Design review of the part shown in the three views and the two pictorial views. Dimensions are in mm from the part's minimum x, y and z. A direction names the side the tool comes from. Coordinates: 2 decimals unless noted, no trailing zeros. Write each loop counter-clockwise with the first axis right and the second up, starting at its lowest first coordinate (ties: lowest second). Pieces come first, ordered by that corner, then holes.
Q1. For the marked faces 4 and 5, list the 3-axis set-ups (+Z, -Z, +X, -X, +Y, -Y) from which the entire face can be reached by the end or side of a thin tool; tool diameter is ignored.
Q2. The part is to be moulded in two halves that separate along Z. For the marked faces 1, 2 and 3, say which applies: released by +Z, released by -Z, zero draft, split by the parting line, or undercut.
Q3. Take a section at C-C, the plane x = 1.25. Write out the cut boundary in (y, z), plus the area to 4 significant figures.
Q4. For pin 1 Ø5 at (x, z) = (4.5, 19) entering from -Y; pin 2 Ø4 at (y, z) = (9.5, 27) entering from +X, all flat-tipped, find the tip position at first contact; note any pin that passes through.
Q5. Take a section at B-B, the plane y = 18.5. Write out the cut boundary in (x, z).
Q6. For L1, parallel to Z at x = 8.75, y = 38; L2, parallel to Y at x = 2.5, z = 2, list the stretches that pass through material, from the lowest coordinate up.
Q7. Take a section at A-A, the plane z = 27. Write out the cut boundary in (x, y).
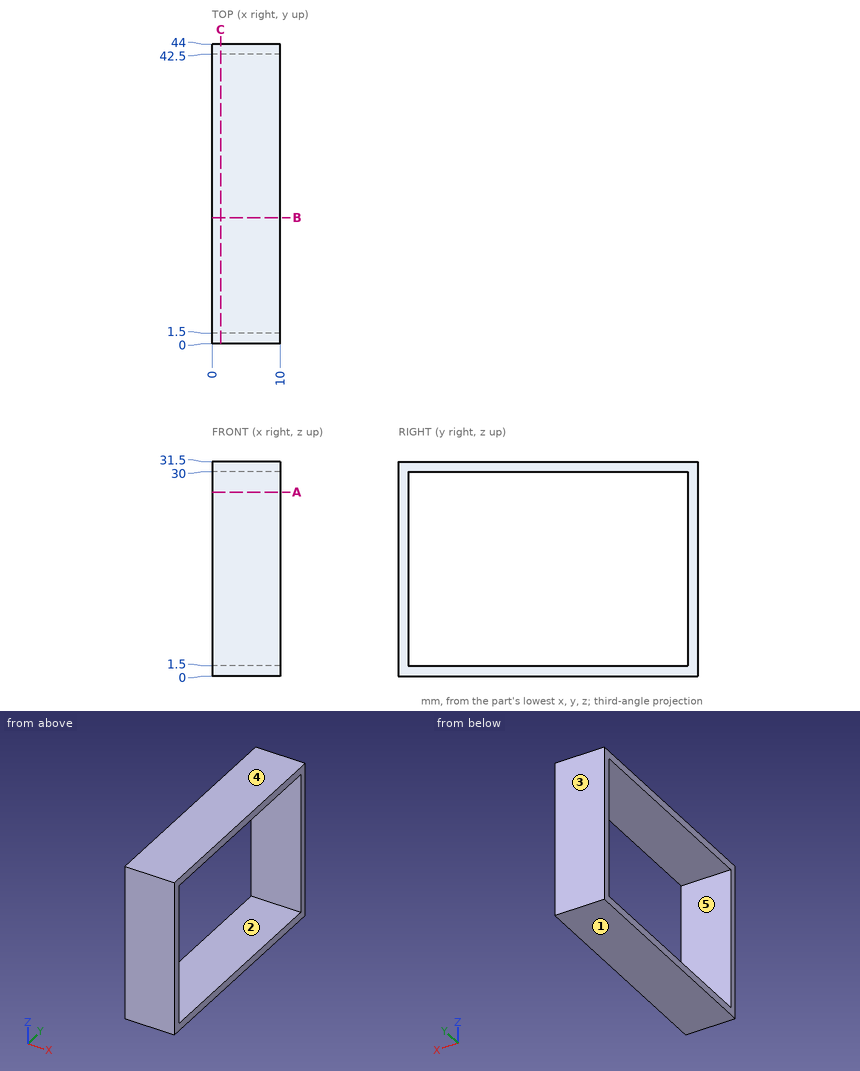
Responses:
1. face 4: +Z, +X, -X, +Y, -Y
1. face 5: +X, -X
2. face 1: released by -Z
2. face 2: undercut
2. face 3: zero draft
3. outline: (0, 0) - (44, 0) - (44, 31.5) - (0, 31.5) - close; hole (1.5, 1.5) - (42.5, 1.5) - (42.5, 30) - (1.5, 30) - close
3. area: 217.5 mm2
4. pin 1: stops at y = 0
4. pin 2: passes through
5. outline: (0, 0) - (10, 0) - (10, 1.5) - (0, 1.5) - close; (0, 30) - (10, 30) - (10, 31.5) - (0, 31.5) - close
6. L1: z = 0 to 1.5, 30 to 31.5
6. L2: y = 0 to 1.5, 42.5 to 44
7. outline: (0, 0) - (10, 0) - (10, 1.5) - (0, 1.5) - close; (0, 42.5) - (10, 42.5) - (10, 44) - (0, 44) - close
